The listing builds one solid part. Answer for the finished solid, in the listing's coordinates (mm). A direction names the side the tool comes from. Coordinates: 2 decimals unless noted, no trailing zeros. Write each loop counter-clockwise with the first axis right and the second up, starting at its lowest first coordinate (ties: lowest second). Pieces come first, ordered by that corner, then holes. Notation, with made-up numbers: M 39,76.5 L 73,76.5 A23 cw 73,99.5 Z; hole C -13,71.25 d8. An arc over 180 degrees is marked long. Write item = value, one per line. Start each with the question number.
```python
from build123d import *

# Parameters (mm, degrees)
SALIENTE_EXTRUIR1_DEPTH    = 3.81
S_LIDO_MOVER_COPIAR2_ANGLE = 180
SALIENTE_EXTRUIR2_START    = -25.4
CROQUIS2_R                 = 9.5
SALIENTE_EXTRUIR2_DEPTH    = 146.05
MATRIZL1_COUNT             = 3
MATRIZL1_PITCH             = 146.05
S_LIDO_MOVER_COPIAR3_ANGLE = 120
S_LIDO_MOVER_COPIAR4_ANGLE = 120
CROQUIS3_R                 = 9.5
SALIENTE_EXTRUIR3_DEPTH    = 27.94


with BuildPart() as part:
    # Croquis1 → Saliente-Extruir1 (new body, symmetric)
    with BuildSketch(Plane(origin=(0, 0, 0), x_dir=(1, 0, 0), z_dir=(0, 1, 0))):
        with BuildLine():
            Line((-5.499261314, 15.875), (-10.998522628, 6.35))
            ThreePointArc((-10.998522628, 6.35), (0, -12.7), (10.998522628, 6.35))
            Line((10.998522628, 6.35), (5.499261314, 15.875))
            ThreePointArc((5.499261314, 15.875), (0, 19.05), (-5.499261314, 15.875))
        make_face()
    extrude(amount=SALIENTE_EXTRUIR1_DEPTH, both=True)


with BuildPart() as body_2:
    # S_lido-Mover_Copiar1: copy of part
    add(part.part.moved(Location((0, 60.96, 0))))


with BuildPart() as body_2_1:
    # S_lido-Mover_Copiar2: moved
    add(body_2.part.rotate(Axis((0, 0, 0), (0, 1, 0)), S_LIDO_MOVER_COPIAR2_ANGLE))


with BuildPart() as part_1:
    add(part.part)

    add(body_2_1.part)  # Saliente-Extruir2 merges body 2
    # Croquis2 → Saliente-Extruir2 (add)
    with BuildSketch(Plane(origin=(0, 0, 0), x_dir=(1, 0, 0), z_dir=(0, 1, 0)).offset(SALIENTE_EXTRUIR2_START)):
        Circle(CROQUIS2_R)
    extrude(amount=SALIENTE_EXTRUIR2_DEPTH)


with BuildPart() as matrizl1_1:
    # MatrizL1: pattern copy
    add(part_1.part.moved(Location(Vector(0, 1, 0) * (1 * MATRIZL1_PITCH))))


with BuildPart() as matrizl1_2:
    # MatrizL1: pattern copy
    add(part_1.part.moved(Location(Vector(0, 1, 0) * (2 * MATRIZL1_PITCH))))


with BuildPart() as matrizl1_1_1:
    # S_lido-Mover_Copiar3: moved
    add(matrizl1_1.part.rotate(Axis((0, 0, 0), (0, 1, 0)), S_LIDO_MOVER_COPIAR3_ANGLE))


with BuildPart() as matrizl1_2_1:
    # S_lido-Mover_Copiar4: moved
    add(matrizl1_2.part.rotate(Axis((0, 0, 0), (0, -1, 0)), S_LIDO_MOVER_COPIAR4_ANGLE))


with BuildPart() as part_2:
    add(part_1.part)

    # Croquis3 → Saliente-Extruir3 (add)
    with BuildSketch(Plane.XZ.offset(25.4)):
        Circle(CROQUIS3_R)
    extrude(amount=SALIENTE_EXTRUIR3_DEPTH)


with BuildPart() as matrizl1_2_2:
    add(matrizl1_2_1.part)

    # Combinar1: union MatrizL1_1, part
    add(matrizl1_1_1.part)
    add(part_2.part)


solid = matrizl1_2_2.part
```
1. For faces 1 (the face through (-2.059, 384.419, 9.274)), 2 (the face through (-13.71, 146.1, -1.65)), 3 (the face through (13.8, 292.2, -1.5)), 4 (the face through (-7, 349.25, -7)), 5 (the face through (13.71, 207.06, 1.65)), determine the directions among +Z, -Z, +X, -X, +Y, -Y from which every point of the face is accessible in a straight line to the end or side of a thin tool.
2. The part is cut by section A-A, the plane y = 274.5. Write down the section's boundary in (x, z).
3. For a pull along Y with two mould halves and no side action, classify faces 6 (the face through (8.2, 61, 11.2)), 7 (the face through (-7, 356.87, -7)), 8 (the face through (1, -3.81, -10)), 9 (the face through (-11.18, 207.063, 6.025)) as pulls with the +Y half, pulls with the -Y half, needs draft (parallel to the pull), parting line crosses it, or undercut.
4. Each of these flat-tipped pins is pushed along its axis until it touches: pin 1 (8 mm diameter, centred on x = 2, y = 320.5, fed in from -Z); pin 2 (10 mm diameter, centred on x = -7.5, y = 104.5, fed in from -Z); pin 3 (3 mm diameter, centred on x = -9.5, y = 171, fed in from -Z). Where does it stop, or does it pass through?
5. Straight lines are drawn through the part: L1, parallel to Y at x = 8, z = -7; L2, parallel to Y at x = 4, z = 14.5; L3, parallel to Z at x = 7, y = 374.5. For each, find the intervals that lie inside material, in ascending order. Write a range as [from, to].
Solution:
q1.face_1 = +Y
q1.face_2 = -Z, -X, -Y
q1.face_3 = -Z, +X, +Y
q1.face_4 = none
q1.face_5 = +Z, +X, -Y
q2.outline = C 0,0 d19
q3.face_6 = needs draft
q3.face_7 = pulls with the +Y half
q3.face_8 = pulls with the -Y half
q3.face_9 = undercut
q4.pin_1 = -9.5
q4.pin_2 = -9.17
q4.pin_3 = -5.12
q5.L1 = [-3.81, 3.81], [57.15, 64.77], [142.24, 149.86], [203.2, 210.82], [288.29, 295.91], [349.25, 356.87]
q5.L2 = [57.15, 64.77]
q5.L3 = [-6.42, 6.42]
